from build123d import *

# Parameters (mm, degrees)
SKETCH_2_W          = 82
SKETCH_2_H          = 54
SKETCH_2_R          = 1.35
SKETCH_2_R_2        = 1.05
EXTRUDE_1_DEPTH     = 3
SKETCH_3_R          = 3
SKETCH_3_R_2        = 1.35
EXTRUDE_2_DEPTH     = 5.2
SKETCH_4_W          = 82
SKETCH_4_H          = 3
EXTRUDE_3_DEPTH     = 40
SKETCH_5_R          = 1.35
SKETCH_5_R_2        = 1.1
SKETCH_5_R_3        = 8
CUT_EXTRUDE_1_DEPTH = 4
SKETCH_6_W          = 54
SKETCH_6_H          = 43
SKETCH_6_R          = 1.35
SKETCH_6_R_2        = 1.05
EXTRUDE_4_DEPTH     = 3
SKETCH_7_R          = 3.35
SKETCH_7_R_2        = 1.35
EXTRUDE_5_DEPTH     = 1.6
SKETCH_8_W          = 8
SKETCH_8_H          = 8
SKETCH_8_R          = 1.05
EXTRUDE_6_DEPTH     = 3
SKETCH_9_W          = 8
SKETCH_9_H          = 8
SKETCH_9_R          = 1.05
EXTRUDE_7_DEPTH     = 3
SKETCH_11_R         = 1.05
CUT_EXTRUDE_2_DEPTH = 5
CHAMFER_1_SIZE      = 1
CHAMFER_2_SIZE      = 6
CHAMFER_3_SIZE      = 1.6


# Some blends are built 0.0001 mm under size
with BuildPart() as part:
    # 草图2 → 凸台-拉伸1 (new body)
    with BuildSketch(Plane(origin=(0, 0, 0), x_dir=(1, 0, 0), z_dir=(0, 1, 0))):
        Rectangle(SKETCH_2_W, SKETCH_2_H)
        with Locations(Location((0, 13.75, 0), (0, 0, 270))):
            Circle(SKETCH_2_R, mode=Mode.SUBTRACT)
        with Locations(Location((0, -13.75, 0), (0, 0, 90))):
            Circle(SKETCH_2_R, mode=Mode.SUBTRACT)
        with Locations(Location((38.5, -24.5, 0), (0, 0, 270))):
            Circle(SKETCH_2_R_2, mode=Mode.SUBTRACT)
    extrude(amount=EXTRUDE_1_DEPTH)

    # 草图3 → 凸台-拉伸2 (add)
    # profile 1 of 2: a face of its own
    with BuildSketch(Plane(origin=(0, 3, 0), x_dir=(1, 0, 0), z_dir=(0, 1, 0))):
        with Locations(Location((0, 13.75, 0), (0, 0, 90))):
            Circle(SKETCH_3_R)
        with Locations(Location((0, 13.75, 0), (0, 0, 270))):
            Circle(SKETCH_3_R_2, mode=Mode.SUBTRACT)
    # profile 2 of 2: a face of its own
    with BuildSketch(Plane(origin=(0, 3, 0), x_dir=(1, 0, 0), z_dir=(0, 1, 0))):
        with Locations(Location((0, -13.75, 0), (0, 0, 90))):
            Circle(SKETCH_3_R)
        with Locations(Location((0, -13.75, 0), (0, 0, 90))):
            Circle(SKETCH_3_R_2, mode=Mode.SUBTRACT)
    extrude(amount=EXTRUDE_2_DEPTH)

    # 草图4 → 凸台-拉伸3 (add)
    with BuildSketch(Plane(origin=(0, 3, 0), x_dir=(1, 0, 0), z_dir=(0, 1, 0))):
        with Locations((0, 25.5)):
            Rectangle(SKETCH_4_W, SKETCH_4_H)
    extrude(amount=EXTRUDE_3_DEPTH)

    # 草图5 → 切除-拉伸1 (cut)
    with BuildSketch(Plane(origin=(0, 0, -27), x_dir=(-1, 0, 0), z_dir=(0, 0, -1))):
        with Locations((-13.423393759, 11.25)):
            Circle(SKETCH_5_R)
        with Locations((-9.526279442, 13.5)):
            Circle(SKETCH_5_R_2)
        with Locations((13.423393759, 11.25)):
            Circle(SKETCH_5_R)
        with Locations((9.526279442, 13.5)):
            Circle(SKETCH_5_R_2)
        with Locations((0, 30)):
            Circle(SKETCH_5_R_2)
        with Locations((0, 34.5)):
            Circle(SKETCH_5_R)
        with Locations((0, 19)):
            Circle(SKETCH_5_R_3)
    extrude(amount=-CUT_EXTRUDE_1_DEPTH, mode=Mode.SUBTRACT)

    # 草图6 → 凸台-拉伸4 (add)
    with BuildSketch(Plane.ZY.offset(41)):
        with Locations((0, 21.5)):
            Rectangle(SKETCH_6_W, SKETCH_6_H)
        with Locations((-10.25, 22)):
            Circle(SKETCH_6_R, mode=Mode.SUBTRACT)
        with Locations(Location((12.25, 22, 0), (0, 0, 180))):
            Circle(SKETCH_6_R, mode=Mode.SUBTRACT)
        with Locations((24.5, 40.5)):
            Circle(SKETCH_6_R_2, mode=Mode.SUBTRACT)
    extrude(amount=-EXTRUDE_4_DEPTH)

    # 草图7 → 凸台-拉伸5 (add)
    # profile 1 of 2: a face of its own
    with BuildSketch(Plane(origin=(-38, 0, 0), x_dir=(0, 0, -1), z_dir=(1, 0, 0))):
        with Locations(Location((-12.25, 22, 0), (0, 0, 180))):
            Circle(SKETCH_7_R)
        with Locations((-12.25, 22)):
            Circle(SKETCH_7_R_2, mode=Mode.SUBTRACT)
    # profile 2 of 2: a face of its own
    with BuildSketch(Plane(origin=(-38, 0, 0), x_dir=(0, 0, -1), z_dir=(1, 0, 0))):
        with Locations(Location((10.25, 22, 0), (0, 0, 180))):
            Circle(SKETCH_7_R)
        with Locations(Location((10.25, 22, 0), (0, 0, 180))):
            Circle(SKETCH_7_R_2, mode=Mode.SUBTRACT)
    extrude(amount=EXTRUDE_5_DEPTH)

    # 草图8 → 凸台-拉伸6 (add)
    with BuildSketch(Plane(origin=(0, 40, 0), x_dir=(1, 0, 0), z_dir=(0, 1, 0))):
        with Locations((-37, 23)):
            Rectangle(SKETCH_8_W, SKETCH_8_H)
        with Locations(Location((-35.5, 21.5, 0), (0, 0, 270))):
            Circle(SKETCH_8_R, mode=Mode.SUBTRACT)
    extrude(amount=-EXTRUDE_6_DEPTH)

    # 草图9 → 凸台-拉伸7 (add)
    with BuildSketch(Plane.XY.offset(24)):
        with Locations((-37, 4)):
            Rectangle(SKETCH_9_W, SKETCH_9_H)
        with Locations((-35.5, 5.5)):
            Circle(SKETCH_9_R, mode=Mode.SUBTRACT)
    extrude(amount=-EXTRUDE_7_DEPTH)

    # 草图11 → 切除-拉伸2 (cut)
    with BuildSketch(Plane(origin=(0, 0, -27), x_dir=(-1, 0, 0), z_dir=(0, 0, -1))):
        with Locations((-38.5, 40.5)):
            Circle(SKETCH_11_R)
    extrude(amount=-CUT_EXTRUDE_2_DEPTH, mode=Mode.SUBTRACT)

    # 倒角1
    chamfer_1_edges = [part.edges().sort_by_distance(p)[0] for p in [
        (-38, 41.5, -24),
        (-33, 38.5, -19),
        (-38, 3, -1.5),
        (-33, 8, 22.5),
        (-41, 43, 0),
        (41, 43, -25.5),
        (0, 43, -27),
        (0, 0, 27),
        (-41, 0, 0),
        (0, 0, -27),
        (41, 0, 0),
        (41, 1.5, 27),
        (-41, 21.5, 27),
        (-41, 21.5, -27),
        (41, 21.5, -27),
        (1.5, 3, -24),
        (-39.5, 43, 27),
        (-38, 3, 25.5),
        (-38, 20, -24),
    ]]
    chamfer(chamfer_1_edges, length=CHAMFER_1_SIZE)

    # 倒角2
    # the kernel refuses this chamfer: 6 mm, written as the material it adds along each edge
    with BuildSketch(Plane(origin=(-48.910726879, 37, -12.089273121), x_dir=(0.7068394360706733, 0.027495876610586785, 0.7068394360706736), z_dir=(0.7071067811865476, 0, -0.7071067811865476))) as chamfer_2_piece_1_section:
        Polygon((CHAMFER_2_SIZE * 0.999621916911, CHAMFER_2_SIZE * 0.0274958766106), (-CHAMFER_2_SIZE * 0.0274958766106, CHAMFER_2_SIZE * 0.999621916911), (0, 0), align=None)
    chamfer_2_piece_1 = extrude(amount=32.274409418, mode=Mode.PRIVATE)
    chamfer_2_piece_1 = split(chamfer_2_piece_1, bisect_by=Plane(origin=(-34.186783964, 35.742495362, -19), z_dir=(0, 0, -1)), keep=Keep.TOP, mode=Mode.PRIVATE)
    chamfer_2_piece_1 = split(chamfer_2_piece_1, bisect_by=Plane(origin=(-41, 35.742495362, -20.186783964), z_dir=(1, 0, 0)), keep=Keep.TOP, mode=Mode.PRIVATE)
    chamfer_2_piece_1 = split(chamfer_2_piece_1, bisect_by=Plane(origin=(-33, 35.742495362, -20.186783964), z_dir=(-1, 0, 0)), keep=Keep.TOP, mode=Mode.PRIVATE)
    chamfer_2_piece_1 = split(chamfer_2_piece_1, bisect_by=Plane(origin=(-33.5, 35.742495362, -19.5), z_dir=(-0.7071067811865476, 0, -0.7071067811865476)), keep=Keep.TOP, mode=Mode.PRIVATE)
    chamfer_2_piece_1 = chamfer_2_piece_1 - Plane(origin=(-35.5, 35.742495362, -21.5), x_dir=(0, 0, 1), z_dir=(0, 1, 0)) * Cylinder(1.05, 89, mode=Mode.PRIVATE)
    chamfer_2_piece_1 = split(chamfer_2_piece_1, bisect_by=Plane(origin=(-34.186783964, 35.742495362, -27), z_dir=(0, 0, 1)), keep=Keep.TOP, mode=Mode.PRIVATE)
    add(chamfer_2_piece_1)
    with BuildSketch(Plane(origin=(-48.910726879, 14.910726879, 21), x_dir=(0.7068394360706735, 0.7068394360706735, 0.027495876610586212), z_dir=(0.7071067811865476, -0.7071067811865476, 0))) as chamfer_2_piece_2_section:
        Polygon((CHAMFER_2_SIZE * 0.999621916911, -CHAMFER_2_SIZE * 0.0274958766106), (-CHAMFER_2_SIZE * 0.0274958766106, -CHAMFER_2_SIZE * 0.999621916911), (0, 0), align=None)
    chamfer_2_piece_2 = extrude(amount=32.274409418, mode=Mode.PRIVATE)
    chamfer_2_piece_2 = split(chamfer_2_piece_2, bisect_by=Plane(origin=(-34.186783964, 8, 19.742495362), z_dir=(0, -1, 0)), keep=Keep.TOP, mode=Mode.PRIVATE)
    chamfer_2_piece_2 = split(chamfer_2_piece_2, bisect_by=Plane(origin=(-41, 6.813216036, 19.742495362), z_dir=(1, 0, 0)), keep=Keep.TOP, mode=Mode.PRIVATE)
    chamfer_2_piece_2 = split(chamfer_2_piece_2, bisect_by=Plane(origin=(-33, 6.813216036, 19.742495362), z_dir=(-1, 0, 0)), keep=Keep.TOP, mode=Mode.PRIVATE)
    chamfer_2_piece_2 = split(chamfer_2_piece_2, bisect_by=Plane(origin=(-34.186783964, 0, 19.742495362), z_dir=(0, 1, 0)), keep=Keep.TOP, mode=Mode.PRIVATE)
    chamfer_2_piece_2 = split(chamfer_2_piece_2, bisect_by=Plane(origin=(-33.5, 7.5, 19.742495362), z_dir=(-0.7071067811865438, -0.7071067811865512, 0)), keep=Keep.TOP, mode=Mode.PRIVATE)
    chamfer_2_piece_2 = chamfer_2_piece_2 - Plane(origin=(-35.5, 5.5, 19.742495362), x_dir=(1, 0, 0), z_dir=(0, 0, 1)) * Cylinder(1.05, 89, mode=Mode.PRIVATE)
    add(chamfer_2_piece_2)

    # 倒角3
    chamfer_3_edges = [part.edges().sort_by_distance(p)[0] for p in [
        (-38, 22, 8.9),
        (-38, 22, -13.6),
    ]]
    chamfer(chamfer_3_edges, length=CHAMFER_3_SIZE - 0.0001)  # a hair under: the kernel refuses the full size


solid = part.part
Geometry: final body of the model. Coordinates: model frame, mm. A direction names the side the tool comes from. Round coordinates to 2 decimals unless told otherwise and drop trailing zeros. Loops run counter-clockwise (first coordinate to the right, second up) from the corner with the lowest first, then second, coordinate; pieces in that order, holes last. Notation, with made-up numbers: (52.25, 32.25) - (95.25, 32.25) arc R18 cw to (95.25, 38.25) - close; hole circle Ø1 at (-28.5, 9). An arc over 180 degrees is marked (long way). Write each question's results on one line, items separated by ' | '. Start each with the question number.
1) Access query for faces 1 (the face through (-36.33, 4.86, 21.2)), 2 (the face through (-33, 38, -22)), 3 (the face through (-34.4, 4.5, 17.9)), 4 (the face through (8, 22, -27)). Directions: +Z, -Z, +X, -X, +Y, -Y. A direction counts if a zero-diameter tool reaches every point of the face in a straight line with its end or side. Return the directions, or none.
2) Cut plane D-D on x = 9.5. Return loops of the section in (y, z).
3) Cut plane B-B on y = 22. Count the separate pieces of the cut face and the enclosed holes in it, then the cut area to 3 significant figures.
4) Line query: probe 1 along Z at (x, y) = (-35.5, 37); probe 2 along X at (y, z) = (24, 24); probe 3 along Z at (x, y) = (-35, 19). Output: solid intervals per line, ascending. Write a range as [from, to].
5) First-contact query: P1, Ø18.5, axis at x = 0, y = 19, coming from the +Z side; P2, Ø8, axis at x = 14, z = 9, coming from the -Y side; P3, Ø5, axis at x = 1, z = 14, coming from the +Y side; P4, Ø4.5, axis at y = 22, z = -10.25, coming from the +X side. Flat tips, straight axial feed; report the tip coordinate or a pass-through.
6) Cut plane A-A on x = 30. Return loops of the section in (y, z).
7) Cut plane C-C on x = -35.5. Return loops of the section in (y, z).
8) Mould query, pull axis X, two halves, no side actions, for faces 5 (the face through (-36.4, 22, 14)), 6 (the face through (38.1, 1.48, 25.47)), 7 (the face through (-37, 40, -22)). Classes: released by +X, released by -X, zero draft, split by the parting line, or undercut.
Verdict:
1) face 1: +Z | face 2: +Z, +X, +Y | face 3: none | face 4: -Z, +X, -X, +Y, -Y
2) outline: (0, -26) - (1, -27) - (12.4, -27) - (12.4, -24) - (4, -24) - (3, -23) - (3, 27) - (1, 27) - (0, 26) - close; (14.6, -27) - (42, -27) - (43, -26) - (43, -24) - (14.6, -24) - close
3) separate pieces: 4 | enclosed holes: 0 | area: 355 mm2
4) probe 1: z = [-27, -22.55], [-20.45, -19] | probe 2: x = [-41, -38] | probe 3: z = [-27, -24]
5) P1: stops at z = -24 | P2: stops at y = 0 | P3: stops at y = 8.2 | P4: stops at x = -36.4
6) outline: (0, -26) - (1, -27) - (42, -27) - (43, -26) - (43, -24) - (4, -24) - (3, -23) - (3, 27) - (1, 27) - (0, 26) - close
7) outline: (0, -26) - (1, -27) - (42, -27) - (43, -26) - (43, -24) - (40, -24) - (40, -22.55) - (33.09, -22.55) - (32.06, -24) - (4, -24) - (3, -23) - (3, 16.06) - (4.45, 17.09) - (4.45, 24) - (3, 24) - (3, 27) - (1, 27) - (0, 26) - close; (6.55, 18.57) - (8, 19.6) - (8, 24) - (6.55, 24) - close; (34.57, -20.45) - (40, -20.45) - (40, -19) - (35.6, -19) - close
8) face 5: released by +X | face 6: undercut | face 7: zero draft
